```python
from build123d import *

# Parameters (mm, degrees)
F1_DEPTH = 6.35
F0_W     = 101.6
F0_H     = 12.7
F2_DEPTH = 101.6
F4_D     = 14.2875


with BuildPart() as f1:
    # F0 (on Front) → F1 (new body, symmetric)
    with BuildSketch(Plane.XZ):
        Polygon((101.6, 0), (0, 0), (-228.6, 0), (-254, -25.4), (-254, -152.4), (-25.4, -152.4), (101.6, -25.4), align=None)
    extrude(amount=F1_DEPTH, both=True)

    # F0 (on Front) → F2 (join, symmetric)
    with BuildSketch(Plane.XZ):
        with Locations((50.8, 6.35)):
            Rectangle(F0_W, F0_H)
    extrude(amount=F2_DEPTH, both=True)

    # F4 (through all)
    with Locations(Plane.XY.offset(12.7)):
        with Locations((25.4, 76.2), (76.2, 76.2), (76.2, -76.2), (25.4, -76.2)):
            Hole(F4_D / 2)


solid = f1.part
```
Model file for the job. Use its own axes, mm. A direction names the side the tool comes from. Give positions to 0.01 mm unless a question says otherwise; leave off trailing zeros. Loops run counter-clockwise (first coordinate to the right, second up) from the corner with the lowest first, then second, coordinate; pieces in that order, holes last. Notation, with made-up numbers: (33, -29.5) - (78, -29.5) arc R27 cw to (78, 6.5) - close; hole circle Ø6 at (27, -19.5). An arc over 180 degrees is marked (long way). One line per item, written item: value. Start each with the question number.
1. Which spindle directions (+Z, -Z, +X, -X, +Y, -Y) get a long thin tool onto all of the face, cutting with end or side? Do faces 1 (the cylindrical face through (69.601, -78.936, 6.261)), 2 (the flat face through (50, -55, 0)), 3 (the flat face through (-79, 6.35, -75)). Say none if no direction does.
2. Pull direction X, two halves, no side cores. Call faces 4 (the cylindrical face through (32.537, -75.886, 6.261)), 5 (the flat face through (-113, 0, 0)), 6 (the flat face through (-241.1, -0.1, -12.5)): pulls with the +X half, pulls with the -X half, needs draft (parallel to the pull), parting line crosses it, or undercut.
3. Pin check, flat tips, straight feed: pin 1 (10 mm diameter, centred on y = -11.5, z = 5.5, fed in from -X); pin 2 (8 mm diameter, centred on x = 16.5, z = -84, fed in from +Y); pin 3 (18.5 mm diameter, centred on x = 25.4, y = 76.2, fed in from -Z). Stop position of each tip, or through.
4. Slice it at A-A (x = 76.2). List the corners of the cut face in (y, z), plus the area to 3 significant figures.
5. Slice it at B-B (y = 76.2). List the corners of the cut face in (x, z), plus the area to 3 significant figures.
6. Slice it at C-C (x = 4). List the corners of the cut face in (y, z).
7. Slice it at D-D (z = -118.5). List the corners of the cut face in (x, y).
8. Probe L1, parallel to X at y = -76, z = 5; L2, parallel to Y at x = 76.2, z = 6.5; L3, parallel to Z at x = 87, y = 35.5. List the from-to ranges inside material, lowest first. Write a range as from..to.
Solution:
1. face 1: +Z, -Z
1. face 2: -Z, +X, -X, -Y
1. face 3: -Z, +X, -X, +Y
2. face 4: undercut
2. face 5: needs draft
2. face 6: pulls with the -X half
3. pin 1: stops at x = 0
3. pin 2: stops at y = 6.35
3. pin 3: stops at z = 0
4. outline: (-101.6, 0) - (-83.34, 0) - (-83.34, 12.7) - (-101.6, 12.7) - close; (-69.06, 0) - (-6.35, 0) - (-6.35, -50.8) - (6.35, -50.8) - (6.35, 0) - (69.06, 0) - (69.06, 12.7) - (-69.06, 12.7) - close; (83.34, 0) - (101.6, 0) - (101.6, 12.7) - (83.34, 12.7) - close
4. area: 2,860 mm^2
5. outline: (0, 0) - (18.26, 0) - (18.26, 12.7) - (0, 12.7) - close; (32.54, 0) - (69.06, 0) - (69.06, 12.7) - (32.54, 12.7) - close; (83.34, 0) - (101.6, 0) - (101.6, 12.7) - (83.34, 12.7) - close
5. area: 927 mm^2
6. outline: (-101.6, 0) - (-6.35, 0) - (-6.35, -123) - (6.35, -123) - (6.35, 0) - (101.6, 0) - (101.6, 12.7) - (-101.6, 12.7) - close
7. outline: (-254, -6.35) - (8.5, -6.35) - (8.5, 6.35) - (-254, 6.35) - close
8. L1: x = 0..18.26, 32.54..69.06, 83.34..101.6
8. L2: y = -101.6..-83.34, -69.06..69.06, 83.34..101.6
8. L3: z = 0..12.7
